from build123d import *

# Parameters (mm, degrees)
F1_DEPTH = 5.08
F2_W     = 38.1
F2_H     = 6.35
F3_DEPTH = 30.48
F4_W     = 38.1
F4_H     = 6.35
F4_H_2   = 12.7
F5_DEPTH = 5.08
F7_DEPTH = 40.64
F8_R     = 3.175
F9_DEPTH = 25.4


with BuildPart() as f1:
    # F0 (on Top) → F1 (new body)
    with BuildSketch(Plane.XY):
        Polygon((-77.543311, 10.219596), (-77.543311, 3.869596), (-39.443311, 3.869596), (-39.443311, 10.219596), (-39.443311, 16.569596), (-39.443311, 22.919596), (-77.543311, 22.919596), (-77.543311, 16.569596), align=None)
    extrude(amount=F1_DEPTH)

    # F2 (on face) → F3 (join)
    with BuildSketch(Plane.XY.offset(5.08)):
        with Locations((-58.493311, 19.744596)):
            Rectangle(F2_W, F2_H)
        with Locations((-58.493311, 7.044596)):
            Rectangle(F2_W, F2_H)
    extrude(amount=F3_DEPTH)

    # F4 (on face) → F5 (join)
    with BuildSketch(Plane.XY.offset(35.56)):
        with Locations((-58.493311, 7.044596)):
            Rectangle(F4_W, F4_H)
        with Locations((-58.493311, 16.569596)):
            Rectangle(F4_W, F4_H_2)
    extrude(amount=F5_DEPTH)

    # F6 (on face) → F7 (join, through all)
    with BuildSketch(Plane.XY.offset(40.64)):
        with BuildLine():
            ThreePointArc((-39.443311, 58.479596), (-21.663311, 40.699596), (-39.443311, 22.919596))
            Line((-39.443311, 22.919596), (-39.443311, 3.869596))
            ThreePointArc((-39.443311, 3.869596), (-18.668383, 32.543039), (-28.358519, 66.599833))
            Line((-28.358519, 66.599833), (-30.095377, 67.966251))
            ThreePointArc((-30.095377, 67.966251), (-36.355643, 67.8164), (-39.443311, 62.368493))
            Line((-39.443311, 62.368493), (-39.443311, 58.479596))
        make_face()
        with BuildLine():
            ThreePointArc((-51.803668, 58.497424), (-45.919491, 61.378092), (-39.443311, 62.368493))
            ThreePointArc((-39.443311, 62.368493), (-36.355643, 67.8164), (-30.095377, 67.966251))
            Line((-30.095377, 67.966251), (-34.285495, 71.262692))
            ThreePointArc((-34.285495, 71.262692), (-39.06814, 72.563992), (-43.329022, 70.031807))
            Line((-43.329022, 70.031807), (-51.803668, 58.497424))
        make_face()
        with BuildLine():
            ThreePointArc((-49.514539, 55.352199), (-44.716124, 57.679756), (-39.443311, 58.479596))
            Line((-39.443311, 58.479596), (-39.443311, 62.368493))
            ThreePointArc((-39.443311, 62.368493), (-45.919491, 61.378092), (-51.803668, 58.497424))
            Line((-51.803668, 58.497424), (-49.514539, 55.352199))
        make_face()
    extrude(amount=-F7_DEPTH)

    # F8 (on face) → F9 (cut)
    with BuildSketch(Plane(origin=(0, 22.919596, 0), x_dir=(-1, 0, 0), z_dir=(0, 1, 0))):
        with Locations((64.843311, 20.32)):
            Circle(F8_R)
        with Locations((52.143311, 20.32)):
            Circle(F8_R)
    extrude(amount=-F9_DEPTH, mode=Mode.SUBTRACT)


solid = f1.part
Input: part model. Units: mm. Frame: model coordinates. A direction names the side the tool comes from. Coordinates: 2 decimals unless noted, no trailing zeros. Loops run counter-clockwise (first coordinate to the right, second up) from the corner with the lowest first, then second, coordinate; pieces in that order, holes last.
Q1. Cut plane B-B (z = 20.32). Give the number of separate pieces and of enclosed holes in the cut face, then the cut area to 3 significant figures.
Q2. Set-up query: faces 1 (the face through (-48.97, 19.79, 20.46)), 2 (the face through (-39.443, 13, 21)), 3 (the face through (-59, 22.92, 20)). Return all of +Z, -Z, +X, -X, +Y, -Y with unobstructed straight access to the full face (end or side cutting, diameter ignored); none if empty.
Q3. Cut plane D-D (z = 13). Output: boundary loops of the cut face in (x, y), then the cut area to 3 significant figures.
Q4. Material intervals for line 1 (Y direction, x = -62, z = 23); line 2 (X direction, y = 7, z = 20); line 3 (X direction, y = 19, z = 20), sorted ascending.
Q5. Cut plane A-A (x = -58.5). Output: boundary loops of the cut face in (y, z).
Q6. Draft query along Z for faces 4 (the face through (-59, 16.57, 20)), 5 (the face through (-41, 21, 0)), 6 (the face through (-77.543, 18, 20)). Return one class per face: +Z half, -Z half, draft (parallel to the pull), parting line (faces both ways), or undercut.
Q7. Contact query for flat-ended pins moving along their axis: pin 1 (15 mm diameter, centred on x = -56, z = 17, fed in from +Y); pin 2 (3 mm diameter, centred on y = 12.5, z = 15.5, fed in from -X); pin 3 (1 mm diameter, centred on x = -60, z = 24.5, fed in from +Y); pin 4 (4 mm diameter, centred on x = -64.84, z = 20.32, fed in from -Y). Output: stop coordinate, or through.
Q8. Cut plane C-C (x = -24). Output: boundary loops of the cut face in (y, z).
Working result:
1. separate pieces: 5
1. enclosed holes: 0
1. area: 1,020 mm2
2. face 1: -Y
2. face 2: -X
2. face 3: +Z, -Z, -X
3. outline: (-77.54, 3.87) - (-39.44, 3.87) arc R40.53 ccw to (-28.36, 66.6) - (-30.1, 67.97) - (-34.29, 71.26) arc R6.35 ccw to (-43.33, 70.03) - (-51.8, 58.5) - (-49.51, 55.35) arc R17.78 cw to (-39.44, 58.48) arc R17.78 cw to (-39.44, 22.92) - (-77.54, 22.92) - (-77.54, 16.57) - (-39.44, 16.57) - (-39.44, 10.22) - (-77.54, 10.22) - close
3. area: 1,180 mm2
4. line 1: y = 3.87 to 10.22, 16.57 to 22.92
4. line 2: x = -77.54 to -68, -61.68 to -55.3, -48.98 to -34.49
4. line 3: x = -77.54 to -68, -61.68 to -55.3, -48.98 to -23.67
5. outline: (3.87, 0) - (22.92, 0) - (22.92, 40.64) - (3.87, 40.64) - close; hole (10.22, 5.08) - (16.57, 5.08) - (16.57, 35.56) - (10.22, 35.56) - close
6. face 4: undercut
6. face 5: -Z half
6. face 6: draft
7. pin 1: stops at y = 62.99
7. pin 2: stops at x = -39.44
7. pin 3: stops at y = 22.92
7. pin 4: passes through
8. outline: (18.46, 0) - (31.89, 0) - (31.89, 40.64) - (18.46, 40.64) - close; (49.51, 0) - (60.73, 0) - (60.73, 40.64) - (49.51, 40.64) - close
